from build123d import *

# Parameters (mm, degrees)
BOSS_EXTRUDE1_DEPTH     = 0.6
CHAMFER1_SIZE           = 0.6
CHAMFER1_SIZE_2         = 3.402769092
CUT_EXTRUDE1_DEPTH      = 64.893348637
CUT_EXTRUDE1_DEPTH_BACK = 64.893348637


with BuildPart() as part:
    # Sketch1 → Boss-Extrude1 (new body)
    with BuildSketch(Plane(origin=(0, 0, 0), x_dir=(1, 0, 0), z_dir=(0, 1, 0))):
        Polygon((0, 0), (61, 0), (46, 19), (15, 19), align=None)
    extrude(amount=BOSS_EXTRUDE1_DEPTH)

    # Chamfer1
    # the kernel refuses this chamfer: 3.402769092, 0.6 mm, written as the material it takes off along each edge
    with BuildSketch(Plane(origin=(-8.8422275, 0.6, 0), x_dir=(0, -0.9776715712462579, 0.2101387607674348), z_dir=(1, 0, 0))) as chamfer1_piece_1:
        Polygon((CHAMFER1_SIZE * 0.977671571246, CHAMFER1_SIZE * 0.210138760767), (-CHAMFER1_SIZE_2 * 0.210138760753, CHAMFER1_SIZE_2 * 0.97767157118), (0, 0), align=None)
    extrude(amount=78.684455, mode=Mode.SUBTRACT)

    # Sketch2 → Cut-Extrude1 (cut, two sides: drawn at the far end of the back side and taken through both)
    with BuildSketch(Plane(origin=(0, 0.6, 0), x_dir=(1, 0, 0), z_dir=(0, 1, 0)).offset(-CUT_EXTRUDE1_DEPTH_BACK)):
        with BuildLine():
            Line((25.7, 16.450898266), (25.7, 22.487224665))
            ThreePointArc((25.7, 22.487224665), (27.35, 24.137224665), (29, 22.487224665))
            Line((29, 22.487224665), (29, 16.450898266))
            ThreePointArc((29, 16.450898266), (27.35, 14.800898266), (25.7, 16.450898266))
        make_face()
        with BuildLine():
            Line((32, 16.450898266), (32, 22.487224665))
            ThreePointArc((32, 22.487224665), (33.65, 24.137224665), (35.3, 22.487224665))
            Line((35.3, 22.487224665), (35.3, 16.450898266))
            ThreePointArc((35.3, 16.450898266), (33.65, 14.800898266), (32, 16.450898266))
        make_face()
    extrude(amount=CUT_EXTRUDE1_DEPTH + CUT_EXTRUDE1_DEPTH_BACK, mode=Mode.SUBTRACT)


solid = part.part
For this review, take the finished solid that the model builds, in its own axes (mm). Give positions to 0.01 mm unless a question says otherwise; leave off trailing zeros. Order: outer loops, then holes, each group sorted by start corner. A loop starts at its lowest first (then second) coordinate and runs counter-clockwise, first axis right, second up. Notation, with made-up numbers: (68, 5) - (113, 5) arc R28 cw to (113, 27) - close; hole circle Ø6 at (83, -10.5). An arc over 180 degrees is marked (long way). Answer as a JSON object with one key per item and string values. Group by question number.
Item 1: Wall thickness on line 1 along X through (y, z) = (0.2, -16.25); line 2 along X through (y, z) = (0.4, -17); line 3 along X through (y, z) = (0.3, -4.25): over which ranges is each line inside the solid? List them lowest first.
Item 2: Take a section at C-C on z = -6.5. Give the boundary of the cut face in (x, y), and give its area (3 significant figures).
Item 3: Take a section at A-A on x = 27.35. Give the boundary of the cut face in (y, z), and give its area (3 significant figures).
Item 4: Take a section at B-B on y = 0.35. Give the boundary of the cut face in (x, z), and give its area (3 significant figures).
Item 5: Draft analysis for pull direction X (two halves, no side actions). For faces 1 (the cylindrical face through (27.4, 0.3, -14.8)), 2 (the flat face through (30, 0.6, -11)), 3 (the cylindrical face through (33.7, 0.3, -14.8)), 4 (the flat face through (53.605, 0.296, -9.367)), state which applies: pulls with the +X half, pulls with the -X half, needs draft (parallel to the pull), parting line crosses it, or undercut.
Reported:
{
 "1": {"line 1": "12.83 to 25.71, 28.99 to 32.01, 35.29 to 48.17", "line 2": "13.42 to 25.7, 29 to 32, 35.3 to 47.58", "line 3": "3.36 to 57.64"},
 "2": {"outline": "(5.13, 0) - (55.87, 0) - (55.87, 0.6) - (5.13, 0.6) - close", "area": "30.4 mm^2"},
 "3": {"outline": "(0, -14.8) - (0.6, -14.8) - (0.6, -3.4) - (0, 0) - close", "area": "7.86 mm^2"},
 "4": {"outline": "(1.57, -1.98) - (15, -19) - (25.7, -19) - (25.7, -16.45) arc R1.65 cw to (29, -16.45) - (29, -19) - (32, -19) - (32, -16.45) arc R1.65 cw to (35.3, -16.45) - (35.3, -19) - (46, -19) - (59.43, -1.98) - close", "area": "731 mm^2"},
 "5": {"face 1": "undercut", "face 2": "needs draft", "face 3": "undercut", "face 4": "pulls with the +X half"}
}
